CAD build for the part. Positions are in the model's coordinates, mm. A direction names the side the tool comes from. Give positions to 0.01 mm unless a question says otherwise; leave off trailing zeros. Write each loop counter-clockwise with the first axis right and the second up, starting at its lowest first coordinate (ties: lowest second). Pieces come first, ordered by that corner, then holes. Notation, with made-up numbers: (82.25, 21) -> (114.25, 21) arc R20 ccw to (114.25, 36) -> close; hole circle Ø9 at (6.25, 58.25). An arc over 180 degrees is marked (long way). Answer as a JSON object with one key per item and string values.
```python
from build123d import *

# Parameters (mm, degrees)
SKETCH_W        = 35
SKETCH_H        = 40
PAD_DEPTH       = 5
SKETCH001_W     = 5
SKETCH001_H     = 40
PAD001_DEPTH    = 65
SKETCH002_R     = 15
POCKET_DEPTH    = 35.001
FILLET_R        = 10
FILLET001_R     = 10
FILLET002_R     = 10
SKETCH003_R     = 1.6
POCKET001_DEPTH = 5.001
FILLET003_R     = 1
FILLET004_R     = 1


with BuildPart() as part:
    # Sketch → Pad (new body)
    with BuildSketch(Plane.XY):
        with Locations((-17.5, 20)):
            Rectangle(SKETCH_W, SKETCH_H)
    extrude(amount=PAD_DEPTH)

    # Sketch001 (on Face6 of Pad) → Pad001 (join)
    with BuildSketch(Plane.XY.offset(5)):
        with Locations((-32.5, 20)):
            Rectangle(SKETCH001_W, SKETCH001_H)
        with Locations((-2.5, 20)):
            Rectangle(SKETCH001_W, SKETCH001_H)
    extrude(amount=PAD001_DEPTH)

    # Sketch002 (on Face9 of Pad001) → Pocket (cut, through all)
    with BuildSketch(Plane.YZ):
        with Locations((20, 50)):
            Circle(SKETCH002_R)
    extrude(amount=-POCKET_DEPTH, mode=Mode.SUBTRACT)

    # Fillet
    fillet_edges = [part.edges().sort_by_distance(p)[0] for p in [
        (-32.5, 0, 70),
    ]]
    fillet(fillet_edges, radius=FILLET_R)

    # Fillet001
    fillet001_edges = [part.edges().sort_by_distance(p)[0] for p in [
        (-2.5, 0, 70),
    ]]
    fillet(fillet001_edges, radius=FILLET001_R)

    # Fillet002
    fillet002_edges = [part.edges().sort_by_distance(p)[0] for p in [
        (-32.5, 40, 70),
        (-2.5, 40, 70),
    ]]
    fillet(fillet002_edges, radius=FILLET002_R)

    # Sketch003 (on Face7 of Fillet002) → Pocket001 (cut, through all)
    with BuildSketch(Plane.XY.offset(5)):
        with Locations((-17.5, 30)):
            Circle(SKETCH003_R)
        with Locations((-17.5, 10)):
            Circle(SKETCH003_R)
    extrude(amount=-POCKET001_DEPTH, mode=Mode.SUBTRACT)

    # Fillet003
    fillet003_edges = [part.edges().sort_by_distance(p)[0] for p in [
        (0, 0, 2.5),
        (0, 0, 32.5),
        (0, 2.928932, 67.071068),
        (0, 20, 70),
        (0, 37.071068, 67.071068),
        (0, 40, 32.5),
        (0, 40, 2.5),
    ]]
    fillet(fillet003_edges, radius=FILLET003_R)

    # Fillet004
    fillet004_edges = [part.edges().sort_by_distance(p)[0] for p in [
        (-35, 0, 32.5),
        (-35, 0, 2.5),
        (-35, 2.928932, 67.071068),
        (-35, 20, 70),
        (-35, 37.071068, 67.071068),
        (-35, 40, 32.5),
        (-35, 40, 2.5),
    ]]
    fillet(fillet004_edges, radius=FILLET004_R)


solid = part.part
```
1) Mould opens along X. For faces 3 (the flat face through (0, 20, 26)), 4 (the flat face through (-5, 20, 30)), 5 (the cylindrical face through (-31.97, 3.01, 67.15)) say: released by +X, released by -X, zero draft, split by the parting line, or undercut.
Model answer:
{"face 3": "released by +X", "face 4": "undercut", "face 5": "zero draft"}
2) Slice it at D-D (z = 14.5). List the corners of the cut face in (x, y).
Model answer:
{"outline": "(-35, 1) arc R1 ccw to (-34, 0) -> (-30, 0) -> (-30, 40) -> (-34, 40) arc R1 ccw to (-35, 39) -> close; (-5, 0) -> (-1, 0) arc R1 ccw to (0, 1) -> (0, 39) arc R1 ccw to (-1, 40) -> (-5, 40) -> close"}
3) Slice it at B-B (z = 50). List the corners of the cut face in (x, y), then the cut area to 3 significant figures.
Model answer:
{"outline": "(-35, 1) arc R1 ccw to (-34, 0) -> (-30, 0) -> (-30, 5) -> (-35, 5) -> close; (-35, 35) -> (-30, 35) -> (-30, 40) -> (-34, 40) arc R1 ccw to (-35, 39) -> close; (-5, 0) -> (-1, 0) arc R1 ccw to (0, 1) -> (0, 5) -> (-5, 5) -> close; (-5, 35) -> (0, 35) -> (0, 39) arc R1 ccw to (-1, 40) -> (-5, 40) -> close", "area": "99.1 mm2"}
4) Wall check: probe 1 along Y at (x, z) = (-17.5, 1.2); probe 2 along Z at (x, y) = (-1.6, 20); probe 3 along X at (y, z) = (24, 14.5). Give the ranges that are in metal, low to high.
Model answer:
{"probe 1": "y = 0 to 8.4, 11.6 to 28.4, 31.6 to 40", "probe 2": "z = 0 to 35, 65 to 70", "probe 3": "x = -35 to -30, -5 to 0"}
5) Slice it at A-A (x = -17.5). List the corners of the cut face in (y, z), then the cut area to 3 significant figures.
Model answer:
{"outline": "(0, 0) -> (8.4, 0) -> (8.4, 5) -> (0, 5) -> close; (11.6, 0) -> (28.4, 0) -> (28.4, 5) -> (11.6, 5) -> close; (31.6, 0) -> (40, 0) -> (40, 5) -> (31.6, 5) -> close", "area": "168 mm2"}
6) Slice it at C-C (y = 20). List the corners of the cut face in (x, z).
Model answer:
{"outline": "(-35, 0) -> (0, 0) -> (0, 35) -> (-5, 35) -> (-5, 5) -> (-30, 5) -> (-30, 35) -> (-35, 35) -> close; (-35, 65) -> (-30, 65) -> (-30, 70) -> (-34, 70) arc R1 ccw to (-35, 69) -> close; (-5, 65) -> (0, 65) -> (0, 69) arc R1 ccw to (-1, 70) -> (-5, 70) -> close"}
7) 3-axis set-ups, long thin cutter, end or side, ignore diameter. For faces 1 (the flat face through (-32, 20, 70)), 2 (the flat face through (-18, 20, 5)): which of +Z, -Z, +X, -X, +Y, -Y reach the whole face in a straight line?
Model answer:
{"face 1": "+Z, +X, -X, +Y, -Y", "face 2": "+Z, +Y, -Y"}
8) Pin check, flat tips, straight feed: pin 1 (5 mm diameter, centred on x = -17.5, y = 30, fed in from -Z); pin 2 (3.5 mm diameter, centred on x = -17.5, y = 10, fed in from +Z); pin 3 (1.5 mm diameter, centred on y = 7.5, z = 47.5, fed in from +X). Stop position of each tip, or through.
Model answer:
{"pin 1": "stops at z = 0", "pin 2": "stops at z = 5", "pin 3": "passes through"}
